Autodesk Inventor part; units mm, degrees
ref_plane "YZ Plane" through (0, 0, 0) normal (1, 0, 0) x (0, 1, 0)
ref_plane "XZ Plane" through (0, 0, 0) normal (0, 1, 0) x (-1, 0, 0)
ref_plane "XY Plane" through (0, 0, 0) normal (0, 0, 1) x (1, 0, 0)
sketch "Sketch1" plane through (0, 0, 0) normal (0, 0, 1) x (1, 0, 0)
  line L0 (0, 0) -> (275, 0)
  line L1 (275, 0) -> (275, 200)
  line L2 (275, 200) -> (0, 200)
  line L3 (0, 200) -> (0, 0)
  dimension "d0" = 275
  dimension "d1" = 200
extrude "Extrusion1" add sketch "Sketch1" along normal blind 20
sketch "Sketch3" plane through (0, 0, 20) normal (0, 0, 1) x (1, 0, 0)
  line L0 (275, 0) -> (275, 200)
  line L1 (0, 200) -> (275, 200)
  line L2 (275, 200) -> (275, 0)
  line L3 (275, 0) -> (0, 0)
  line L4 (0, 0) -> (0, 200)
  point P0 (0, 0)
extrude "Extrusion3" add sketch "Sketch3" along normal blind 80
sketch "Sketch4" plane through (0, 0, 0) normal (0, -1, 0) x (1, 0, 0)
  circle A0 centre (47.5, 50) radius 17.5
  circle A1 centre (227.5, 50) radius 17.5
  line L0 (47.5, 50) -> (227.5, 50) construction
  line L1 (0, 0) -> (0, 100)
  line L2 (0, 100) -> (275, 100)
  point P0 (0, 50)
  point P1 (137.5, 50)
  point P2 (137.5, 100)
  dimension "d10" = 35
  dimension "d11" = 35
  dimension "d12" = 180
extrude "Extrusion4" cut sketch "Sketch4" against normal blind 100 contours A0
sketch "Sketch5" plane through (0, 200, 0) normal (0, 1, 0) x (1, 0, 0)
  line L0 (275, 0) -> (0, 0)
  line L1 (0, 0) -> (0, -100)
  line L2 (275, -100) -> (0, -100)
  line L3 (275, 0) -> (275, -100)
  line L4 (265, -90) -> (10, -90)
  line L5 (10, -90) -> (10, -10)
  line L6 (10, -10) -> (265, -10)
  line L7 (265, -10) -> (265, -90)
  point P0 (0, 0)
  dimension "d15" = 10
extrude "Extrusion5" cut sketch "Sketch5" against normal blind 190 contours L4 L5 L6 L7
sketch "Sketch6" plane through (0, 0, 0) normal (-1, 0, 0) x (0, 0, 1)
  line L0 (0, 200) -> (100, 200)
  line L1 (0, 200) -> (0, 0)
  line L2 (100, 200) -> (0, 200)
  line L3 (0, 200) -> (0, 190)
  line L4 (0, 190) -> (100, 190)
  line L5 (100, 190) -> (100, 200)
  dimension "d18" = 10
extrude "Extrusion6" cut sketch "Sketch6" against normal through all
sketch "Sketch7" plane through (0, 190, 100) normal (0, 1, 0) x (1, 0, 0)
  line L0 (275, 100) -> (275, 0) construction
  line L1 (0, 100) -> (275, 100) construction
  line L2 (0, 0) -> (0, 100) construction
  line L3 (275, 0) -> (0, 0) construction
  line L4 (265, 10) -> (265, 90) construction
  line L5 (10, 10) -> (265, 10) construction
  line L6 (10, 90) -> (10, 10) construction
  line L7 (265, 90) -> (10, 90) construction
  line L8 (270, 5) -> (270, 95) construction
  line L9 (270, 95) -> (5, 95) construction
  line L10 (5, 95) -> (5, 5) construction
  line L11 (5, 5) -> (270, 5) construction
  circle A0 centre (270, 5) radius 2.5
  circle A1 centre (270, 95) radius 2.5
  circle A2 centre (5, 95) radius 2.5
  circle A3 centre (5, 5) radius 2.5
  point P0 (0, 100)
  dimension "d21" = 5
  dimension "d22" = 5
  dimension "d23" = 5
  dimension "d24" = 5
  dimension "d25" = 5
extrude "Extrusion7" cut sketch "Sketch7" against normal blind 25
sketch "Sketch8" plane through (0, 0, 0) normal (0, -1, 0) x (1, 0, 0)
  line L0 (82, 15) -> (85, 15)
  line L1 (85, 15) -> (85, 35)
  line L2 (85, 35) -> (82, 35)
  line L3 (82, 35) -> (82, 15)
  line L4 (0, 0) -> (0, 100)
  line L5 (0, 0) -> (275, 0)
  line L6 (97, 15) -> (97, 35)
  line L7 (97, 35) -> (94, 35)
  line L8 (94, 35) -> (94, 15)
  line L9 (94, 15) -> (97, 15)
  line L10 (109, 15) -> (109, 35)
  line L11 (109, 35) -> (106, 35)
  line L12 (106, 35) -> (106, 15)
  line L13 (106, 15) -> (109, 15)
  line L14 (121, 15) -> (121, 35)
  line L15 (121, 35) -> (118, 35)
  line L16 (118, 35) -> (118, 15)
  line L17 (118, 15) -> (121, 15)
  line L18 (133, 15) -> (133, 35)
  line L19 (133, 35) -> (130, 35)
  line L20 (130, 35) -> (130, 15)
  line L21 (130, 15) -> (133, 15)
  line L22 (145, 15) -> (145, 35)
  line L23 (145, 35) -> (142, 35)
  line L24 (142, 35) -> (142, 15)
  line L25 (142, 15) -> (145, 15)
  line L26 (157, 15) -> (157, 35)
  line L27 (157, 35) -> (154, 35)
  line L28 (154, 35) -> (154, 15)
  line L29 (154, 15) -> (157, 15)
  line L30 (169, 15) -> (169, 35)
  line L31 (169, 35) -> (166, 35)
  line L32 (166, 35) -> (166, 15)
  line L33 (166, 15) -> (169, 15)
  line L34 (181, 15) -> (181, 35)
  line L35 (181, 35) -> (178, 35)
  line L36 (178, 35) -> (178, 15)
  line L37 (178, 15) -> (181, 15)
  line L38 (193, 15) -> (193, 35)
  line L39 (193, 35) -> (190, 35)
  line L40 (190, 35) -> (190, 15)
  line L41 (190, 15) -> (193, 15)
  line L42 (205, 15) -> (205, 35)
  line L43 (205, 35) -> (202, 35)
  line L44 (202, 35) -> (202, 15)
  line L45 (202, 15) -> (205, 15)
  line L46 (217, 15) -> (217, 35)
  line L47 (217, 35) -> (214, 35)
  line L48 (214, 35) -> (214, 15)
  line L49 (214, 15) -> (217, 15)
  line L50 (229, 15) -> (229, 35)
  line L51 (229, 35) -> (226, 35)
  line L52 (226, 35) -> (226, 15)
  line L53 (226, 15) -> (229, 15)
  line L54 (241, 15) -> (241, 35)
  line L55 (241, 35) -> (238, 35)
  line L56 (238, 35) -> (238, 15)
  line L57 (238, 15) -> (241, 15)
  dimension "d28" = 3
  dimension "d29" = 20
  dimension "d30" = 82
  dimension "d31" = 15
  dimension "d34" = 12
extrude "Extrusion8" cut sketch "Sketch8" against normal through all
sketch "Sketch2" plane through (275, 0, 100) normal (1, 0, 0) x (0, 0, -1)
  circle A0 centre (70, 125) radius 3
  line L0 (100, 0) -> (0, 0)
  line L1 (100, 0) -> (100, 190)
  dimension "d4" = 6
  dimension "d45" = 125
  dimension "d46" = 30
extrude "Extrusion2" cut sketch "Sketch2" against normal through all
properties part number "HA005" material "ABS Plastic"
Check sheet for the modelled part. Datum: model origin and axes. Units: mm. A direction names the side the tool comes from. Round coordinates to 2 decimals unless told otherwise and drop trailing zeros. Order: outer loops, then holes, each group sorted by start corner. A loop starts at its lowest first (then second) coordinate and runs counter-clockwise, first axis right, second up.
1) Section check C-C (z = 24). Give the number of separate pieces and of enclosed holes in the cut face, and give its area (3 significant figures).
2) Section check A-A (y = 158). Record the boundary of the cut face in (x, z), and give its area (3 significant figures).
3) Section check B-B (y = 125). Record the boundary of the cut face in (x, z), and give its area (3 significant figures).
4) Tool access check on faces 1 (the flat face through (82, 5, 25)), 2 (the flat face through (136, 96, 100)), 3 (the flat face through (265, 101, 49)). Record the directions out of +Z, -Z, +X, -X, +Y, -Y that give a thin tool (end or side, any length) a straight path to the whole face; none if there is none.
5) Scan lines: line 1 (Z direction, x = 270, y = 183); line 2 (Z direction, x = 167, y = 140); line 3 (Y direction, x = 270, z = 30). Record each from-to range of solid material in increasing order.
6) Section check D-D (x = 138). Record the boundary of the cut face in (y, z), and give its area (3 significant figures).
Result:
1. separate pieces: 15
1. enclosed holes: 0
1. area: 5,930 mm2
2. outline: (0, 0) - (275, 0) - (275, 100) - (0, 100) - close; hole (10, 10) - (265, 10) - (265, 90) - (10, 90) - close
2. area: 7,100 mm2
3. outline: (0, 0) - (275, 0) - (275, 27) - (265, 27) - (265, 10) - (10, 10) - (10, 27) - (0, 27) - close; (0, 33) - (10, 33) - (10, 90) - (265, 90) - (265, 33) - (275, 33) - (275, 100) - (0, 100) - close
3. area: 6,980 mm2
4. face 1: +Y, -Y
4. face 2: +Z, +X, -X, +Y, -Y
4. face 3: +Y
5. line 1: z = 0 to 2.5, 7.5 to 92.5, 97.5 to 100
5. line 2: z = 0 to 10, 90 to 100
5. line 3: y = 0 to 122, 128 to 190
6. outline: (0, 0) - (190, 0) - (190, 10) - (10, 10) - (10, 90) - (190, 90) - (190, 100) - (0, 100) - close
6. area: 4,600 mm2
